Design review of the part shown in the three views and the two pictorial views. Dimensions are in mm from the part's minimum x, y and z. Round coordinates to 2 decimals unless told otherwise and drop trailing zeros. Order: outer loops, then holes, each group sorted by start corner. A loop starts at its lowest first (then second) coordinate and runs counter-clockwise, first axis right, second up.
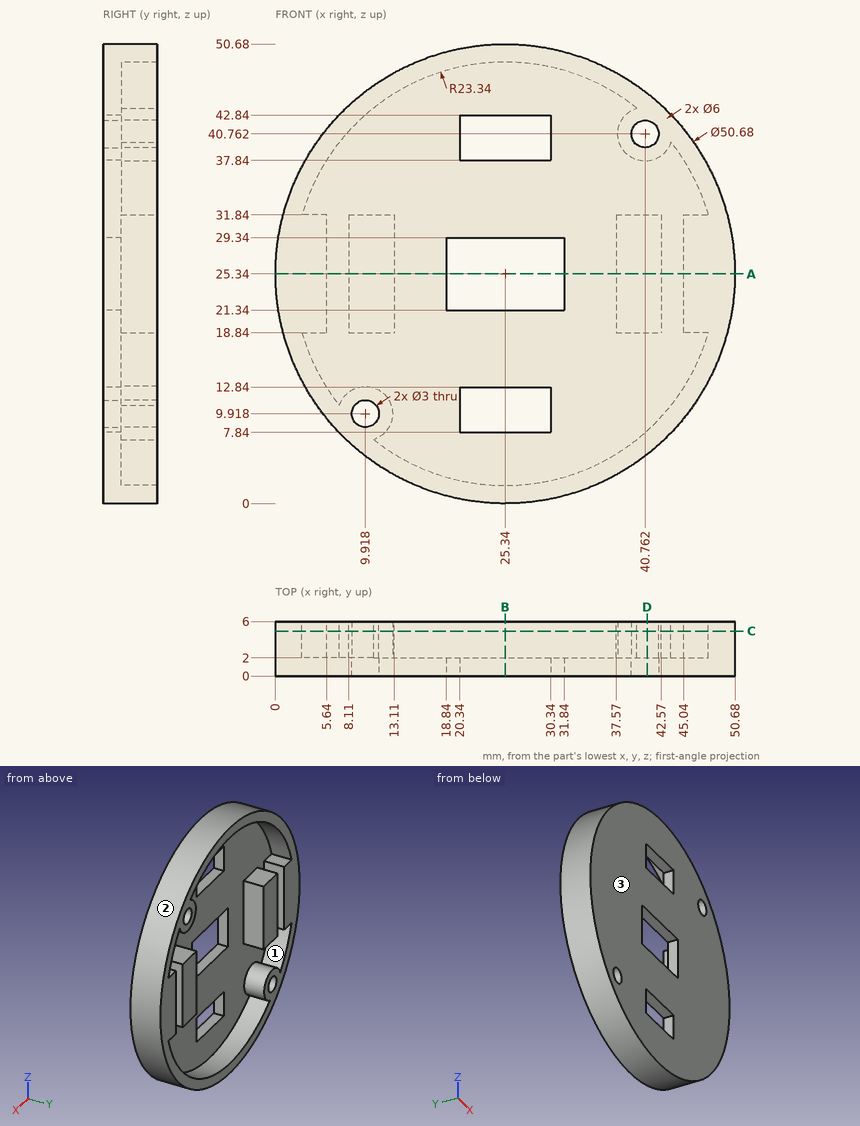
(1) To check wall thickness, follow probe 1 along X at (y, z) = (3.8, 25.5); probe 2 along Z at (x, y) = (40, 2.4); probe 3 along X at (y, z) = (0.4, 25). State the ranges of each line that lie inside material, in increasing order.
Data:
probe 1: x = 0 to 5.64, 8.11 to 13.11, 37.57 to 42.57, 45.04 to 50.68
probe 2: z = 4.67 to 7.18, 18.84 to 31.84, 37.86 to 39.47, 42.05 to 46.01
probe 3: x = 0 to 18.84, 31.84 to 50.68
(2) Consider section B-B (x = 25.34). Write out the cut boundary in (y, z), and give its area (3 significant figures).
Data:
outline: (0, 0) - (6, 0) - (6, 2) - (2, 2) - (2, 7.84) - (0, 7.84) - close; (0, 12.84) - (2, 12.84) - (2, 21.34) - (0, 21.34) - close; (0, 29.34) - (2, 29.34) - (2, 37.84) - (0, 37.84) - close; (0, 42.84) - (2, 42.84) - (2, 48.68) - (6, 48.68) - (6, 50.68) - (0, 50.68) - close
area: 81.4 mm2
(3) Insertion check: pin 1 (2 mm diameter, centred on x = 11.5, y = 5, fed in from +Z); pin 2 (1.6 mm diameter, centred on x = 27.5, y = 1.5, fed in from +Z); pin 3 (0.6 mm diameter, centred on x = 25, y = 1, fed in from +Z); pin 4 (2.5 mm diameter, centred on x = 40.76, z = 40.76, fed in from -Y). Each pin has a flat end and moves straight along its axis. Give the tip position at first contact, or say it passes through.
Data:
pin 1: stops at z = 47.19
pin 2: stops at z = 50.64
pin 3: stops at z = 50.68
pin 4: passes through
(4) Draft analysis for pull direction X (two halves, no side actions). For the marked faces 1, 2 and 3, state which applies: pulls with the +X half, pulls with the -X half, needs draft (parallel to the pull), parting line crosses it, or undercut.
Data:
face 1: undercut
face 2: parting line crosses it
face 3: needs draft
(5) Consider section C-C (y = 4.95). Write out the cut boundary in (x, z).
Data:
outline: circle Ø50.68 at (25.34, 25.34); (8.11, 18.84) - (13.11, 18.84) - (13.11, 31.84) - (8.11, 31.84) - close; (37.57, 18.84) - (42.57, 18.84) - (42.57, 31.84) - (37.57, 31.84) - close; hole (2.92, 18.84) arc R23.34 ccw to (7.06, 10.83) arc R3 cw (long way) to (10.83, 7.06) arc R23.34 ccw to (47.76, 18.84) - (45.04, 18.84) - (45.04, 31.84) - (47.76, 31.84) arc R23.34 ccw to (43.62, 39.85) arc R3 cw (long way) to (39.85, 43.62) arc R23.34 ccw to (2.92, 31.84) - (5.64, 31.84) - (5.64, 18.84) - close; hole circle Ø3 at (9.92, 9.92); hole circle Ø3 at (40.76, 40.76)
(6) Consider section D-D (x = 41). Write out the cut boundary in (y, z).
Data:
outline: (0, 5.42) - (6, 5.42) - (6, 8.03) - (2, 8.03) - (2, 18.84) - (6, 18.84) - (6, 31.84) - (2, 31.84) - (2, 37.77) - (6, 37.77) - (6, 39.28) - (0, 39.28) - close; (0, 42.24) - (6, 42.24) - (6, 45.26) - (0, 45.26) - close
(7) Consider section A-A (z = 25.34). Write out the cut boundary in (x, y), and give its area (3 significant figures).
Data:
outline: (0, 0) - (18.84, 0) - (18.84, 2) - (13.11, 2) - (13.11, 6) - (8.11, 6) - (8.11, 2) - (5.64, 2) - (5.64, 6) - (0, 6) - close; (31.84, 0) - (50.68, 0) - (50.68, 6) - (45.04, 6) - (45.04, 2) - (42.57, 2) - (42.57, 6) - (37.57, 6) - (37.57, 2) - (31.84, 2) - close
area: 160 mm2
